```python
from build123d import *

# Parameters (mm, degrees)
SKETCH1_W           = 70
SKETCH1_H           = 19
SKETCH1_R           = 1.65
BOSS_EXTRUDE1_DEPTH = 3
SKETCH2_R           = 3
CUT_EXTRUDE1_DEPTH  = 3
FILLET2_R           = 9
SKETCH3_R           = 1.65
SKETCH3_R_2         = 3
BOSS_EXTRUDE2_DEPTH = 5.5
FILLET3_R           = 9


with BuildPart() as part:
    # Sketch1 → Boss-Extrude1 (new body)
    with BuildSketch(Plane.XY):
        with Locations((25, 0)):
            Rectangle(SKETCH1_W, SKETCH1_H)
        with Locations((0, 7)):
            Circle(SKETCH1_R, mode=Mode.SUBTRACT)
        with Locations((7, 0)):
            Circle(SKETCH1_R, mode=Mode.SUBTRACT)
        with Locations((0, -7)):
            Circle(SKETCH1_R, mode=Mode.SUBTRACT)
        with Locations((-7, 0)):
            Circle(SKETCH1_R, mode=Mode.SUBTRACT)
    extrude(amount=BOSS_EXTRUDE1_DEPTH)

    # Sketch2 → Cut-Extrude1 (cut)
    with BuildSketch(Plane.XY.offset(3)):
        Circle(SKETCH2_R)
    extrude(amount=-CUT_EXTRUDE1_DEPTH, mode=Mode.SUBTRACT)

    # Fillet2
    fillet2_edges = [part.edges().sort_by_distance(p)[0] for p in [
        (-10, -9.5, 1.5),
        (-10, 9.5, 1.5),
    ]]
    fillet(fillet2_edges, radius=FILLET2_R)

    # Sketch3 → Boss-Extrude2 (add)
    with BuildSketch(Plane.XY.offset(3)):
        with BuildLine():
            Line((-10, 0.5), (-10, -0.5))
            ThreePointArc((-10, -0.5), (-7.363961031, -6.863961031), (-1, -9.5))
            Line((-1, -9.5), (10, -9.5))
            Line((10, -9.5), (10, 9.5))
            Line((10, 9.5), (-1, 9.5))
            ThreePointArc((-1, 9.5), (-7.363961031, 6.863961031), (-10, 0.5))
        make_face()
        with Locations((0, 7)):
            Circle(SKETCH3_R, mode=Mode.SUBTRACT)
        with Locations((-7, 0)):
            Circle(SKETCH3_R, mode=Mode.SUBTRACT)
        with Locations((0, -7)):
            Circle(SKETCH3_R, mode=Mode.SUBTRACT)
        Circle(SKETCH3_R_2, mode=Mode.SUBTRACT)
        with Locations((7, 0)):
            Circle(SKETCH3_R, mode=Mode.SUBTRACT)
    extrude(amount=BOSS_EXTRUDE2_DEPTH)

    # Fillet3
    fillet3_edges = [part.edges().sort_by_distance(p)[0] for p in [
        (10, -9.5, 5.75),
        (10, 9.5, 5.75),
    ]]
    fillet(fillet3_edges, radius=FILLET3_R)


solid = part.part
```
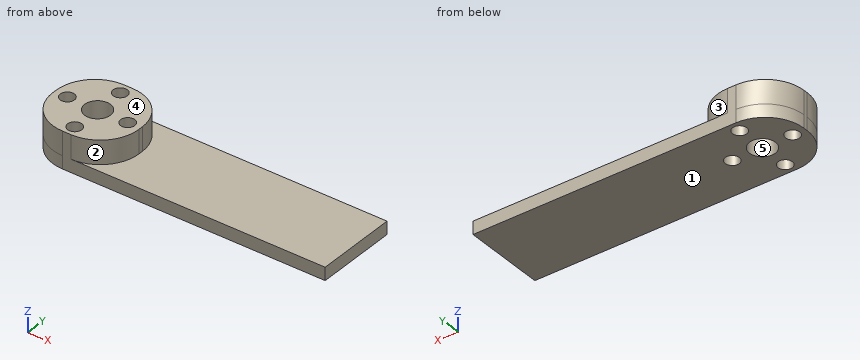
Geometry check sheet. Reference: the model listing, model coordinates, mm. Face numbers are marked on the shaded views. A direction names the side the tool comes from. Round coordinates to 2 decimals unless told otherwise and drop trailing zeros. Order: outer loops, then holes, each group sorted by start corner. A loop starts at its lowest first (then second) coordinate and runs counter-clockwise, first axis right, second up. Notation, with made-up numbers: (71.25, 54) - (95.25, 54) arc R23 cw to (95.25, 93) - close; hole circle Ø9 at (-26.5, -20.75). An arc over 180 degrees is marked (long way). Use a Markdown table: item, result. Add a question column.
1) Mould release check, pull along X, two halves, no side actions. Record for the marked faces 3, 4 and 5: released by +X, released by -X, zero draft, split by the parting line, or undercut.
2) Set-up check for the marked faces 1 and 2: record each of +Z, -Z, +X, -X, +Y, -Y from which the full face is reachable in a straight line by a thin tool's end or side.
3) Gauge pin test, flat ends, axial feed: P1, Ø2, axis at x = 25.5, y = -2.5, coming from the +Z side; P2, Ø0.8, axis at y = 0, z = 6, coming from the +X side. Record the tip position at first contact, or that the pin passes through.
4) Section check D-D (x = 7). Record the cut outline in (y, z), then the cut area to 3 significant figures.
5) Section check B-B (y = 6). Record the cut outline in (x, z), then the cut area to 3 significant figures.
6) Section check C-C (z = 6.25). Record the cut outline in (x, y).
7) Thickness scan on line 1 along Y through (x, z) = (0, 6.75); line 2 along Z through (x, y) = (38.5, -4); line 3 along X through (y, z) = (-8.5, 4.5). Record the ranges inside material, lowest first.
8) Section check A-A (x = 0). Record the cut outline in (y, z), then the cut area to 3 significant figures.
Established:
| question | item | result |
|---|---|---|
| 1 | face 3 | released by +X |
| 1 | face 4 | zero draft |
| 1 | face 5 | undercut |
| 2 | face 1 | -Z, +X, -X, +Y, -Y |
| 2 | face 2 | +Z, +X, -Y |
| 3 | P1 | z = 3 |
| 3 | P2 | x = 10 |
| 4 | outline | (-9.5, 0) - (-1.65, 0) - (-1.65, 8.5) - (-7.21, 8.5) - (-7.21, 3) - (-9.5, 3) - close; (1.65, 0) - (9.5, 0) - (9.5, 3) - (7.21, 3) - (7.21, 8.5) - (1.65, 8.5) - close |
| 4 | area | 108 mm2 |
| 5 | outline | (-8.12, 0) - (-1.31, 0) - (-1.31, 8.5) - (-8.12, 8.5) - close; (1.31, 0) - (60, 0) - (60, 3) - (8.12, 3) - (8.12, 8.5) - (1.31, 8.5) - close |
| 5 | area | 271 mm2 |
| 6 | outline | (-10, -0.5) arc R9 ccw to (-1, -9.5) - (1, -9.5) arc R9 ccw to (10, -0.5) - (10, 0.5) arc R9 ccw to (1, 9.5) - (-1, 9.5) arc R9 ccw to (-10, 0.5) - close; hole circle Ø3.3 at (-7, 0); hole circle Ø6 at (0, 0); hole circle Ø3.3 at (0, -7); hole circle Ø3.3 at (0, 7); hole circle Ø3.3 at (7, 0) |
| 7 | line 1 | -9.5 to -8.65, -5.35 to -3, 3 to 5.35, 8.65 to 9.5 |
| 7 | line 2 | 0 to 3 |
| 7 | line 3 | -5.12 to -0.69, 0.69 to 5.12 |
| 8 | outline | (-9.5, 0) - (-8.65, 0) - (-8.65, 8.5) - (-9.5, 8.5) - close; (-5.35, 0) - (-3, 0) - (-3, 8.5) - (-5.35, 8.5) - close; (3, 0) - (5.35, 0) - (5.35, 8.5) - (3, 8.5) - close; (8.65, 0) - (9.5, 0) - (9.5, 8.5) - (8.65, 8.5) - close |
| 8 | area | 54.4 mm2 |
